The listing builds one solid part. Answer for the finished solid, in the listing's coordinates (mm). Face numbers are marked on the shaded views. A direction names the side the tool comes from. Coordinates: 2 decimals unless noted, no trailing zeros. Order: outer loops, then holes, each group sorted by start corner. A loop starts at its lowest first (then second) coordinate and runs counter-clockwise, first axis right, second up. Notation, with made-up numbers: M 42.5,61 L 95.5,61 A19 cw 95.5,69 Z; hole C 78,-8.75 d1. An arc over 180 degrees is marked long. One line per item, written item: value. Start each with the question number.
Q1. Each of these flat-tipped pins is pushed along its axis until it touches: pin 1 Ø10 at (x, y) = (-37, 35) entering from -Z; pin 2 Ø10 at (x, z) = (-19.05, -12.7) entering from +Y (3 decimals); pin 3 Ø8.5 at (x, z) = (-45.72, 0) entering from +Y; pin 4 Ø5.5 at (x, z) = (31.75, -12.7) entering from -Y. Where does it stop, or does it pass through?
Q2. For the marked faces 1 and 2, determine the directions among +Z, -Z, +X, -X, +Y, -Y from which every point of the face is accessible in a straight line to the end or side of a thin tool.
Q3. The part is cut by section A-A on x = 51. Give the vertices of the cut face in (y, z) (3 decimals).
Q4. Determine the mould class of the marked faces 3 and 4 for opening direction X: pulls with the +X half, pulls with the -X half, needs draft (parallel to the pull), parting line crosses it, or undercut.
Q5. The part is cut by section B-B on y = 96. Give the vertices of the cut face in (x, z) (3 decimals).
Q6. Straight lines are drawn through the part: line 1 along Y through (x, z) = (-49, -5.5) (3 decimals); line 2 along X through (y, z) = (107.5, 2) (3 decimals); line 3 along Y through (x, z) = (-3.5, -14.75) (3 decimals). For each, find the intervals that lie inside material, in ascending order. Write a range as [from, to].
Q7. The part is cut by section C-C on x = -63.5. Give the number of separate pieces and of enclosed holes in the cut face, then the cut area to 3 significant figures.
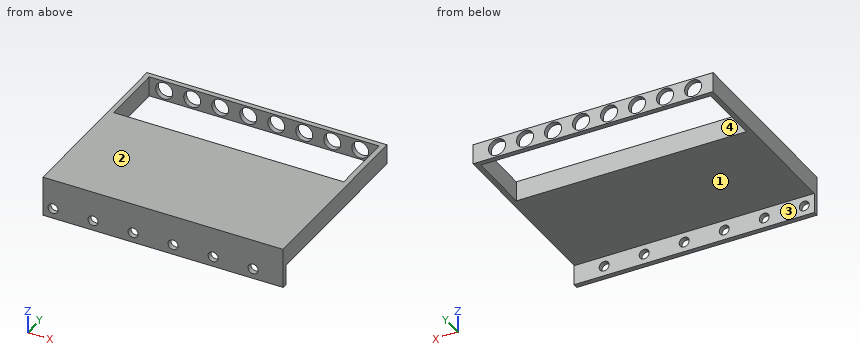
```python
from build123d import *

# Parameters (mm, degrees)
SKETCH1_W           = 152.4
SKETCH1_H           = 12.7
BOSS_EXTRUDE1_DEPTH = 76.2
SKETCH2_R           = 3.175
BOSS_EXTRUDE4_DEPTH = 3.175
BOSS_EXTRUDE5_DEPTH = 12.7
CUT_EXTRUDE1_REACH  = 145.964
SKETCH4_R           = 5.3975


with BuildPart() as part:
    # Sketch1 → Boss-Extrude1 (new body)
    with BuildSketch(Plane(origin=(0, 0, 0), x_dir=(1, 0, 0), z_dir=(0, 1, 0))):
        Rectangle(SKETCH1_W, SKETCH1_H)
    extrude(amount=BOSS_EXTRUDE1_DEPTH)

    # Sketch2 → Boss-Extrude4 (add)
    with BuildSketch(Plane(origin=(0, 0, 0), x_dir=(1, 0, 0), z_dir=(0, 1, 0))):
        Polygon((-76.2, 12.7), (-76.2, 6.35), (76.2, 6.35), (76.2, 19.05), (-76.2, 19.05), align=None)
        with Locations(Location((-69.85, 12.7, 0), (0, 0, 270))):
            Circle(SKETCH2_R, mode=Mode.SUBTRACT)
        with Locations(Location((-44.45, 12.7, 0), (0, 0, 270))):
            Circle(SKETCH2_R, mode=Mode.SUBTRACT)
        with Locations(Location((-19.05, 12.7, 0), (0, 0, 270))):
            Circle(SKETCH2_R, mode=Mode.SUBTRACT)
        with Locations(Location((6.35, 12.7, 0), (0, 0, 270))):
            Circle(SKETCH2_R, mode=Mode.SUBTRACT)
        with Locations(Location((31.75, 12.7, 0), (0, 0, 270))):
            Circle(SKETCH2_R, mode=Mode.SUBTRACT)
        with Locations(Location((57.15, 12.7, 0), (0, 0, 270))):
            Circle(SKETCH2_R, mode=Mode.SUBTRACT)
    extrude(amount=BOSS_EXTRUDE4_DEPTH)

    # Sketch3 → Boss-Extrude5 (add)
    with BuildSketch(Plane.XY.offset(6.35)):
        Polygon((-76.2, 76.2), (-76.2, 120.65), (76.2, 120.65), (76.2, 76.2), (73.025, 76.2), (73.025, 117.475), (-73.025, 117.475), (-73.025, 76.2), align=None)
    extrude(amount=-BOSS_EXTRUDE5_DEPTH)

    # Sketch4 → Cut-Extrude1 (cut, up to next)
    with BuildSketch(Plane(origin=(0, 120.65, 0), x_dir=(1, 0, 0), z_dir=(0, 1, 0)), mode=Mode.PRIVATE) as cut_extrude1_sk1:
        with Locations(Location((-63.5, 0, 0), (0, 0, 270))):
            Circle(SKETCH4_R)
    cut_extrude1_tool1 = extrude(cut_extrude1_sk1.sketch, amount=-CUT_EXTRUDE1_REACH, mode=Mode.PRIVATE) & part.part
    # Sketch4 → Cut-Extrude1 (cut, up to next)
    with BuildSketch(Plane(origin=(0, 120.65, 0), x_dir=(1, 0, 0), z_dir=(0, 1, 0)), mode=Mode.PRIVATE) as cut_extrude1_sk2:
        with Locations(Location((-45.72, 0, 0), (0, 0, 270))):
            Circle(SKETCH4_R)
    cut_extrude1_tool2 = extrude(cut_extrude1_sk2.sketch, amount=-CUT_EXTRUDE1_REACH, mode=Mode.PRIVATE) & part.part
    # Sketch4 → Cut-Extrude1 (cut, up to next)
    with BuildSketch(Plane(origin=(0, 120.65, 0), x_dir=(1, 0, 0), z_dir=(0, 1, 0)), mode=Mode.PRIVATE) as cut_extrude1_sk3:
        with Locations(Location((-27.94, 0, 0), (0, 0, 270))):
            Circle(SKETCH4_R)
    cut_extrude1_tool3 = extrude(cut_extrude1_sk3.sketch, amount=-CUT_EXTRUDE1_REACH, mode=Mode.PRIVATE) & part.part
    # Sketch4 → Cut-Extrude1 (cut, up to next)
    with BuildSketch(Plane(origin=(0, 120.65, 0), x_dir=(1, 0, 0), z_dir=(0, 1, 0)), mode=Mode.PRIVATE) as cut_extrude1_sk4:
        with Locations(Location((-10.16, 0, 0), (0, 0, 270))):
            Circle(SKETCH4_R)
    cut_extrude1_tool4 = extrude(cut_extrude1_sk4.sketch, amount=-CUT_EXTRUDE1_REACH, mode=Mode.PRIVATE) & part.part
    # Sketch4 → Cut-Extrude1 (cut, up to next)
    with BuildSketch(Plane(origin=(0, 120.65, 0), x_dir=(1, 0, 0), z_dir=(0, 1, 0)), mode=Mode.PRIVATE) as cut_extrude1_sk5:
        with Locations(Location((7.62, 0, 0), (0, 0, 270))):
            Circle(SKETCH4_R)
    cut_extrude1_tool5 = extrude(cut_extrude1_sk5.sketch, amount=-CUT_EXTRUDE1_REACH, mode=Mode.PRIVATE) & part.part
    # Sketch4 → Cut-Extrude1 (cut, up to next)
    with BuildSketch(Plane(origin=(0, 120.65, 0), x_dir=(1, 0, 0), z_dir=(0, 1, 0)), mode=Mode.PRIVATE) as cut_extrude1_sk6:
        with Locations(Location((25.4, 0, 0), (0, 0, 270))):
            Circle(SKETCH4_R)
    cut_extrude1_tool6 = extrude(cut_extrude1_sk6.sketch, amount=-CUT_EXTRUDE1_REACH, mode=Mode.PRIVATE) & part.part
    # Sketch4 → Cut-Extrude1 (cut, up to next)
    with BuildSketch(Plane(origin=(0, 120.65, 0), x_dir=(1, 0, 0), z_dir=(0, 1, 0)), mode=Mode.PRIVATE) as cut_extrude1_sk7:
        with Locations(Location((43.18, 0, 0), (0, 0, 270))):
            Circle(SKETCH4_R)
    cut_extrude1_tool7 = extrude(cut_extrude1_sk7.sketch, amount=-CUT_EXTRUDE1_REACH, mode=Mode.PRIVATE) & part.part
    # Sketch4 → Cut-Extrude1 (cut, up to next)
    with BuildSketch(Plane(origin=(0, 120.65, 0), x_dir=(1, 0, 0), z_dir=(0, 1, 0)), mode=Mode.PRIVATE) as cut_extrude1_sk8:
        with Locations(Location((60.96, 0, 0), (0, 0, 270))):
            Circle(SKETCH4_R)
    cut_extrude1_tool8 = extrude(cut_extrude1_sk8.sketch, amount=-CUT_EXTRUDE1_REACH, mode=Mode.PRIVATE) & part.part
    add(cut_extrude1_tool1.solids().sort_by_distance((-63.5, 120.65, 0))[0], mode=Mode.SUBTRACT)
    add(cut_extrude1_tool2.solids().sort_by_distance((-45.72, 120.65, 0))[0], mode=Mode.SUBTRACT)
    add(cut_extrude1_tool3.solids().sort_by_distance((-27.94, 120.65, 0))[0], mode=Mode.SUBTRACT)
    add(cut_extrude1_tool4.solids().sort_by_distance((-10.16, 120.65, 0))[0], mode=Mode.SUBTRACT)
    add(cut_extrude1_tool5.solids().sort_by_distance((7.62, 120.65, 0))[0], mode=Mode.SUBTRACT)
    add(cut_extrude1_tool6.solids().sort_by_distance((25.4, 120.65, 0))[0], mode=Mode.SUBTRACT)
    add(cut_extrude1_tool7.solids().sort_by_distance((43.18, 120.65, 0))[0], mode=Mode.SUBTRACT)
    add(cut_extrude1_tool8.solids().sort_by_distance((60.96, 120.65, 0))[0], mode=Mode.SUBTRACT)


solid = part.part
```
Output:
1. pin 1: stops at z = -6.35
1. pin 2: stops at y = 3.175
1. pin 3: stops at y = 76.2
1. pin 4: passes through
2. face 1: -Z, +X, -X, +Y
2. face 2: +Z, +X, -X, +Y, -Y
3. outline: M 0,-19.05 L 3.175,-19.05 L 3.175,-6.35 L 76.2,-6.35 L 76.2,6.35 L 0,6.35 Z; M 117.475,-6.35 L 120.65,-6.35 L 120.65,6.35 L 117.475,6.35 Z
4. face 3: needs draft
4. face 4: undercut
5. outline: M -76.2,-6.35 L -73.025,-6.35 L -73.025,6.35 L -76.2,6.35 Z; M 73.025,-6.35 L 76.2,-6.35 L 76.2,6.35 L 73.025,6.35 Z
6. line 1: y = [0, 76.2], [117.475, 120.65]
6. line 2: x = [-76.2, -73.025], [73.025, 76.2]
6. line 3: y = [0, 3.175]
7. separate pieces: 3
7. enclosed holes: 0
7. area: 1,010 mm^2
